Geometry check sheet. Reference: the model listing, model coordinates, mm. A direction names the side the tool comes from. Coordinates: 2 decimals unless noted, no trailing zeros. Write each loop counter-clockwise with the first axis right and the second up, starting at its lowest first coordinate (ties: lowest second). Pieces come first, ordered by that corner, then holes.
from build123d import *

# Parameters (mm, degrees)
CYLINDER001_R     = 1.6
CYLINDER001_DEPTH = 4
CYLINDER002_R     = 2.5
CYLINDER002_DEPTH = 16
CYLINDER_R        = 3.5
CYLINDER_DEPTH    = 8
FILLET_R          = 1


with BuildPart() as hole:
    # Cylinder001 → Cylinder001 (new body)
    with BuildSketch(Plane.XY.offset(6)):
        Circle(CYLINDER001_R)
    extrude(amount=CYLINDER001_DEPTH)


with BuildPart() as thread:
    # Cylinder002 → Cylinder002 (new body)
    with BuildSketch(Plane.XY.offset(-15)):
        Circle(CYLINDER002_R)
    extrude(amount=CYLINDER002_DEPTH)


with BuildPart() as obj1:
    # Cylinder → Cylinder (new body)
    with BuildSketch(Plane.XY):
        Circle(CYLINDER_R)
    extrude(amount=CYLINDER_DEPTH)

    # Fusion: union thread
    add(thread.part)

    # Cut: cut hole
    add(hole.part, mode=Mode.SUBTRACT)

    # Fillet
    fillet_edges = [obj1.edges().sort_by_distance(p)[0] for p in [
        (-3.5, 0, 8),
    ]]
    fillet(fillet_edges, radius=FILLET_R)


solid = obj1.part
1. Gauge pin test, flat ends, axial feed: pin 1 Ø4 at (x, z) = (2, -8) entering from -Y; pin 2 Ø1 at (x, z) = (2, -12) entering from -Y. Record the tip position at first contact, or that the pin passes through.
Computed values:
pin 1: stops at y = -2.5
pin 2: stops at y = -2
2. Thickness scan on line 1 along Y through (x, z) = (0, 6.9); line 2 along Y through (x, z) = (0, 7.4); line 3 along Z through (x, y) = (-0.75, -0.25). Record the ranges inside material, lowest first.
Computed values:
line 1: y = -3.5 to -1.6, 1.6 to 3.5
line 2: y = -3.42 to -1.6, 1.6 to 3.42
line 3: z = -15 to 6
3. Sectioned sample at A-A, the plane x = 0. Record the boundary of the cut face in (y, z), and give its area (3 significant figures).
Computed values:
outline: (-3.5, 0) - (-2.5, 0) - (-2.5, -15) - (2.5, -15) - (2.5, 0) - (3.5, 0) - (3.5, 7) arc R1 ccw to (2.5, 8) - (1.6, 8) - (1.6, 6) - (-1.6, 6) - (-1.6, 8) - (-2.5, 8) arc R1 ccw to (-3.5, 7) - close
area: 124 mm2
4. Access from +Z, -Z, +X, -X, +Y, -Y to the whole of each face (thin tool, end or side, straight path). Record for faces 1 (the cylindrical face through (-1.27, -0.97, 6.99)), 2 (the cylindrical face through (-0.54, -2.44, -7.6)), 3 (the flat face through (0, -2, 8)).
Computed values:
face 1: +Z
face 2: -Z
face 3: +Z, +X, -X, +Y, -Y
5. Sectioned sample at C-C, the plane z = -6.75. Record the boundary of the cut face in (x, y), and give its area (3 significant figures).
Computed values:
outline: circle Ø5 at (0, 0)
area: 19.6 mm2
6. Draft check along X on faces 4 (the cylindrical face through (3.233, -1.341, 3.451)), 5 (the flat face through (0, 0, 6)), 6 (the flat face through (2, -2, 0)). Enter one of: released by +X, released by -X, zero draft, split by the parting line, or undercut.
Computed values:
face 4: split by the parting line
face 5: undercut
face 6: zero draft
